Autodesk Inventor part; units mm, degrees
ref_plane "YZ Plane" through (0, 0, 0) normal (1, 0, 0) x (0, 1, 0)
ref_plane "XZ Plane" through (0, 0, 0) normal (0, 1, 0) x (-1, 0, 0)
ref_plane "XY Plane" through (0, 0, 0) normal (0, 0, 1) x (1, 0, 0)
sketch "Sketch1" plane through (0, 0, 0) normal (1, 0, 0) x (0, 1, 0)
  line L0 (0, 0) -> (25.4, 0)
  line L1 (25.4, 0) -> (25.4, -787.4)
  line L2 (25.4, -787.4) -> (0, -787.4)
  line L3 (0, -787.4) -> (0, 0)
  dimension "d0" = 787.4
  dimension "d1" = 25.4
extrude "Extrusion1" add sketch "Sketch1" along normal blind 25.4
sketch "Sketch2" plane through (0, 0, 0) normal (0, 0, 1) x (1, 0, 0)
  line L0 (3.175, 3.175) -> (22.225, 3.175)
  line L1 (22.225, 3.175) -> (22.225, 22.225)
  line L2 (22.225, 22.225) -> (3.175, 22.225)
  line L3 (3.175, 22.225) -> (3.175, 3.175)
  line L4 (0, 25.4) -> (25.4, 25.4)
  line L5 (0, 0) -> (0, 25.4)
  dimension "d4" = 3.175
  dimension "d5" = 3.175
  dimension "d6" = 19.05
  dimension "d7" = 19.05
extrude "Extrusion2" cut sketch "Sketch2" against normal blind 787.4
sketch "Sketch3" plane through (0, 0, 0) normal (0, 0, 1) x (1, 0, 0)
  line L0 (-24.3318, 33.3766) -> (65.9681, 33.3766)
  line L1 (65.9681, 33.3766) -> (65.9681, -31.7467)
  line L2 (65.9681, -31.7467) -> (-24.3318, -31.7467)
  line L3 (-24.3318, -31.7467) -> (-24.3318, 33.3766)
  point P0 (0, 0)
extrude "Extrusion3" cut sketch "Sketch3" against normal blind 50.8
properties part number "1by1by31" material "Aluminum 6061"
For this review, take the finished solid that the model builds, in its own axes (mm). A direction names the side the tool comes from. Round coordinates to 2 decimals unless told otherwise and drop trailing zeros. Write each loop counter-clockwise with the first axis right and the second up, starting at its lowest first coordinate (ties: lowest second). Pieces come first, ordered by that corner, then holes.
1) Insertion check: pin 1 Ø8 at (y, z) = (17.5, -710.5) entering from -X. The pin has a flat end and moves straight along its axis. Give the tip position at first contact, or say it passes through.
Answer below:
pin 1: stops at x = 0
2) Machinability: for faces 1 (the face through (25.4, 13, -414)), 2 (the face through (22.225, 13, -414)), which of the approach directions +Z, -Z, +X, -X, +Y, -Y give a long, thin tool a straight path to every point of the face, cutting with its end or side? Answer none if there is none.
Answer below:
face 1: +Z, -Z, +X, +Y, -Y
face 2: +Z, -Z
3) Mouldability with a two-part tool opening along Y and no side actions: class faces 3 (the face through (3.175, 13, -414)), 4 (the face through (13, 0, -424)), 5 (the face through (13, 2, -787.4)), 6 (the face through (13, 25.4, -414)) as +Y half, -Y half, draft (parallel to the pull), parting line (faces both ways), or undercut.
Answer below:
face 3: undercut
face 4: -Y half
face 5: draft
face 6: +Y half
4) For line 1 along X through (y, z) = (9.25, -90) (3 decimals), list the stretches that pass through material, from the lowest coordinate up.
Answer below:
line 1: x = 0 to 3.175, 22.225 to 25.4
5) Take a section at C-C on z = -512.5. Give the boundary of the cut face in (x, y) (3 decimals), then the cut area to 3 significant figures.
Answer below:
outline: (0, 0) - (25.4, 0) - (25.4, 25.4) - (0, 25.4) - close; hole (3.175, 3.175) - (22.225, 3.175) - (22.225, 22.225) - (3.175, 22.225) - close
area: 282 mm2
6) Take a section at A-A on x = 7. Give the boundary of the cut face in (y, z) (3 decimals).
Answer below:
outline: (0, -787.4) - (3.175, -787.4) - (3.175, -50.8) - (0, -50.8) - close; (22.225, -787.4) - (25.4, -787.4) - (25.4, -50.8) - (22.225, -50.8) - close
